Here's how the part is built. I have some questions about the finished solid (model axes, mm). A direction names the side the tool comes from. Coordinates: 2 decimals unless noted, no trailing zeros. Answer as CSV lines item,"result". Start each with the question number.
Item 1: I need wall thicknesses on line 1 (Y direction, x = 124, z = -7.75); line 2 (Z direction, x = 262.5, y = -14.1); line 3 (Y direction, x = 200, z = 0.5). Which ranges of each line are inside material? Lowest first, please.
Item 2: On a 3-axis mill with a long thin cutter (end or side, diameter ignored), from which of +Z, -Z, +X, -X, +Y, -Y can I reach the whole of each face in a straight line? I mean faces 4 (the face through (7, -6, 0)), 5 (the face through (510.5, 7, 0)). Say none if no direction works.
Item 3: Imagine slicing it at A-A on x = 362.5. Count the separate pieces of the cut face and the enclosed holes in it, and give its area (3 significant figures).
Item 4: We'd pull the mould along Z, two halves only. Please class faces 1 (the face through (-510.5, 7, 0)), 2 (the face through (7, 11, 0)), 3 (the face through (7, 0, 15)): pulls with the +Z half, pulls with the -Z half, needs draft (parallel to the pull), parting line crosses it, or undercut.
Item 5: I'm going to push flat-ended pins straight in: pin 1 (1.6 mm diameter, centred on x = -114.5, z = 10.5, fed in from -Y); pin 2 (1.5 mm diameter, centred on x = -402, z = 6, fed in from +Y); pin 3 (4 mm diameter, centred on x = -148, z = 0, fed in from -Y). Where does each tip first touch, or does it pass through?
from build123d import *

# Parameters (mm, degrees)
SKETCH_1_W             = 23.5
SKETCH_1_H             = 12
EXTRUDE_1_DEPTH        = 510.5
HOLE_WIZARD_M6_1_D     = 5
HOLE_WIZARD_M6_1_DEPTH = 19
HOLE_WIZARD_M6_1_TIP   = 1.502151548
HOLE_WIZARD_M6_2_D     = 5
HOLE_WIZARD_M6_2_DEPTH = 19
HOLE_WIZARD_M6_2_TIP   = 1.502151548
HOLE_WIZARD_M6_3_D     = 5
HOLE_WIZARD_M6_3_DEPTH = 17
HOLE_WIZARD_M6_3_TIP   = 1.502151548
SKETCH_9_R             = 4.5
CUT_EXTRUDE_1_DEPTH    = 512.600674355
SKETCH_10_R            = 4.5
CUT_EXTRUDE_2_DEPTH    = 512.600674355
HOLE_WIZARD_M4_1_D     = 3.3
HOLE_WIZARD_M4_1_DEPTH = 11.5
HOLE_WIZARD_M4_1_TIP   = 0.991420021
HOLE_WIZARD_M4_2_D     = 3.3
HOLE_WIZARD_M4_2_DEPTH = 11.5
HOLE_WIZARD_M4_2_TIP   = 0.991420021


with BuildPart() as part:
    # Sketch 1 → Extrude 1 (new, symmetric)
    with BuildSketch(Plane(origin=(0, 0, 0), x_dir=(0, 0, -1), z_dir=(1, 0, 0))):
        Polygon((-15, 15), (-11.5, 15), (-11.5, 13.5), (-11, 13.5), (-11, 12), (-9.5, 12), (-9.5, 15), (-8, 15), (-8, 12.5), (-5, 12.5), (-5, 15), (5, 15), (5, 12.5), (8, 12.5), (8, 15), (9.5, 15), (9.5, 12), (11, 12), (11, 13.5), (11.5, 13.5), (11.5, 15), (15, 15), (15, 8), (12.5, 8), (12.5, 5), (15, 5), (15, -5), (12.5, -5), (12.5, -8), (15, -8), (15, -15), (11.5, -15), (11.5, -13.5), (11, -13.5), (11, -12), (9.5, -12), (9.5, -15), (8, -15), (8, -12.5), (5, -12.5), (5, -15), (-5, -15), (-5, -12.5), (-8, -12.5), (-8, -15), (-9.5, -15), (-9.5, -12), (-11, -12), (-11, -13.5), (-11.5, -13.5), (-11.5, -15), (-15, -15), align=None)
        with BuildLine():
            Line((12, -10.5), (12, -8.5))
            ThreePointArc((12, -8.5), (11.853553391, -8.146446609), (11.5, -8))
            Line((11.5, -8), (-11.5, -8))
            ThreePointArc((-11.5, -8), (-11.853553391, -8.146446609), (-12, -8.5))
            Line((-12, -8.5), (-12, -10.5))
            ThreePointArc((-12, -10.5), (-11.853553391, -10.853553391), (-11.5, -11))
            Line((-11.5, -11), (11.5, -11))
            ThreePointArc((11.5, -11), (11.853553391, -10.853553391), (12, -10.5))
        make_face(mode=Mode.SUBTRACT)
        with BuildLine():
            Line((-11.5, 11), (11.5, 11))
            ThreePointArc((11.5, 11), (11.853553391, 10.853553391), (12, 10.5))
            Line((12, 10.5), (12, 8.5))
            ThreePointArc((12, 8.5), (11.853553391, 8.146446609), (11.5, 8))
            Line((11.5, 8), (-11.5, 8))
            ThreePointArc((-11.5, 8), (-11.853553391, 8.146446609), (-12, 8.5))
            Line((-12, 8.5), (-12, 10.5))
            ThreePointArc((-12, 10.5), (-11.853553391, 10.853553391), (-11.5, 11))
        make_face(mode=Mode.SUBTRACT)
        Rectangle(SKETCH_1_W, SKETCH_1_H, mode=Mode.SUBTRACT)
    extrude(amount=EXTRUDE_1_DEPTH, both=True)

    # Hole Wizard M6 _1
    with Locations(Plane(origin=(0, -15, 0), x_dir=(-1, 0, 0), z_dir=(0, -1, 0))):
        with Locations((-460.5, 0), (-445.5, 0), (133, 0), (148, 0), (218, 0), (233, 0), (445.5, 0), (460.5, 0)):
            Hole(HOLE_WIZARD_M6_1_D / 2, depth=HOLE_WIZARD_M6_1_DEPTH)
            with Locations((0, 0, -(HOLE_WIZARD_M6_1_DEPTH + HOLE_WIZARD_M6_1_TIP / 2))):  # 118° drill point
                Cone(0, HOLE_WIZARD_M6_1_D / 2, HOLE_WIZARD_M6_1_TIP, mode=Mode.SUBTRACT)

    # Hole Wizard M6 _2
    with Locations(Plane(origin=(0, 0, -15), x_dir=(-1, 0, 0), z_dir=(0, 0, -1))):
        with Locations((460.5, 0), (445.5, 0), (-142.5, 0), (-157.5, 0), (-445.5, 0), (-460.5, 0), (380.5, 0)):
            Hole(HOLE_WIZARD_M6_2_D / 2, depth=HOLE_WIZARD_M6_2_DEPTH)
            with Locations((0, 0, -(HOLE_WIZARD_M6_2_DEPTH + HOLE_WIZARD_M6_2_TIP / 2))):  # 118° drill point
                Cone(0, HOLE_WIZARD_M6_2_D / 2, HOLE_WIZARD_M6_2_TIP, mode=Mode.SUBTRACT)

    # Hole Wizard M6 _3
    with Locations(Plane(origin=(0, -15, 0), x_dir=(-1, 0, 0), z_dir=(0, -1, 0))):
        with Locations((-262.5, 0), (-211.5, 0)):
            Hole(HOLE_WIZARD_M6_3_D / 2, depth=HOLE_WIZARD_M6_3_DEPTH)
            with Locations((0, 0, -(HOLE_WIZARD_M6_3_DEPTH + HOLE_WIZARD_M6_3_TIP / 2))):  # 118° drill point
                Cone(0, HOLE_WIZARD_M6_3_D / 2, HOLE_WIZARD_M6_3_TIP, mode=Mode.SUBTRACT)

    # Sketch 9 → Cut-Extrude 1 (cut, through all)
    with BuildSketch(Plane.XY.offset(15)):
        with Locations((415.5, 0)):
            Circle(SKETCH_9_R)
        with Locations((-422.5, 0)):
            Circle(SKETCH_9_R)
    extrude(amount=-CUT_EXTRUDE_1_DEPTH, mode=Mode.SUBTRACT)

    # Sketch 10 → Cut-Extrude 2 (cut, through all)
    with BuildSketch(Plane(origin=(0, 15, 0), x_dir=(1, 0, 0), z_dir=(0, 1, 0))):
        with Locations(Location((495.5, 0, 0), (0, 0, 270))):
            Circle(SKETCH_10_R)
        with Locations(Location((-78, 0, 0), (0, 0, 270))):
            Circle(SKETCH_10_R)
    extrude(amount=-CUT_EXTRUDE_2_DEPTH, mode=Mode.SUBTRACT)

    # Hole Wizard M4 _1
    with Locations(Plane(origin=(0, 0, -15), x_dir=(-1, 0, 0), z_dir=(0, 0, -1))):
        with Locations((-429.5, 0), (-401.5, 0)):
            Hole(HOLE_WIZARD_M4_1_D / 2, depth=HOLE_WIZARD_M4_1_DEPTH)
            with Locations((0, 0, -(HOLE_WIZARD_M4_1_DEPTH + HOLE_WIZARD_M4_1_TIP / 2))):  # 118° drill point
                Cone(0, HOLE_WIZARD_M4_1_D / 2, HOLE_WIZARD_M4_1_TIP, mode=Mode.SUBTRACT)

    # Hole Wizard M4 _2
    with Locations(Plane(origin=(0, 0, -15), x_dir=(-1, 0, 0), z_dir=(0, 0, -1))):
        with Locations((-343.5, 0)):
            Hole(HOLE_WIZARD_M4_2_D / 2, depth=HOLE_WIZARD_M4_2_DEPTH)
            with Locations((0, 0, -(HOLE_WIZARD_M4_2_DEPTH + HOLE_WIZARD_M4_2_TIP / 2))):  # 118° drill point
                Cone(0, HOLE_WIZARD_M4_2_D / 2, HOLE_WIZARD_M4_2_TIP, mode=Mode.SUBTRACT)


solid = part.part
Responses:
1,line 1,"y = -12.5 to -11, -8 to -6, 6 to 8, 11 to 12.5"
1,line 2,"z = -15 to -11.5, -9.5 to -8, -5 to -2.5, 2.5 to 5, 8 to 9.5, 11.5 to 15"
1,line 3,"y = -15 to -11, -8 to -6, 6 to 8, 11 to 15"
2,face 4,"+X, -X"
2,face 5,"+Z, -Z, +X, +Y, -Y"
3,separate pieces,"1"
3,enclosed holes,"3"
3,area,"408 mm^2"
4,face 1,"needs draft"
4,face 2,"undercut"
4,face 3,"pulls with the +Z half"
5,pin 1,"stops at y = -13.5"
5,pin 2,"stops at y = 12.5"
5,pin 3,"stops at y = 6"
